Part print with two shaded views. Sizes in mm from the minimum x, y, z corner. A direction names the side the tool comes from. Give positions to 0.01 mm unless a question says otherwise; leave off trailing zeros. Loops run counter-clockwise (first coordinate to the right, second up) from the corner with the lowest first, then second, coordinate; pieces in that order, holes last. Notation, with made-up numbers: M 17.5,-7.5 L 47.5,-7.5 A26 cw 47.5,7.5 Z; hole C 47,86.25 d6. An arc over 180 degrees is marked long. Answer as a JSON object with one key per item and string values. Group by question number.
1. Slice it at B-B (z = 10). List the corners of the cut face in (x, y).
2. Drop flat-ended pins along their axis: pin 1 Ø10.5 at (y, z) = (3.5, 11) entering from -X; pin 2 Ø5.5 at (x, z) = (34, 9) entering from +Y; pin 3 Ø4 at (x, y) = (37.5, 17) entering from -Z. Give the stop position or say it passes through.
3. Slice it at C-C (x = 31). List the corners of the cut face in (y, z).
4. Mould opens along Y. For the marked faces 1, 2 and 3 say: released by +Y, released by -Y, zero draft, split by the parting line, or undercut.
5. Slice it at A-A (x = 25). List the corners of the cut face in (y, z).
6. Slice it at D-D (y = 17.75). List the corners of the cut face in (x, z), then the cut area to 3 significant figures.
7. 3-axis set-ups, long thin cutter, end or side, ignore diameter. For the marked faces 4, 5 and 6: which of +Z, -Z, +X, -X, +Y, -Y reach the whole face in a straight line?
8. Drill centre lines: line 1 along Y through (x, z) = (10, 26); line 2 along X through (y, z) = (3.4, 10); line 3 along Y through (x, z) = (20, 26). Where is each one in solid material? Low to high. Write a range as [from, to].
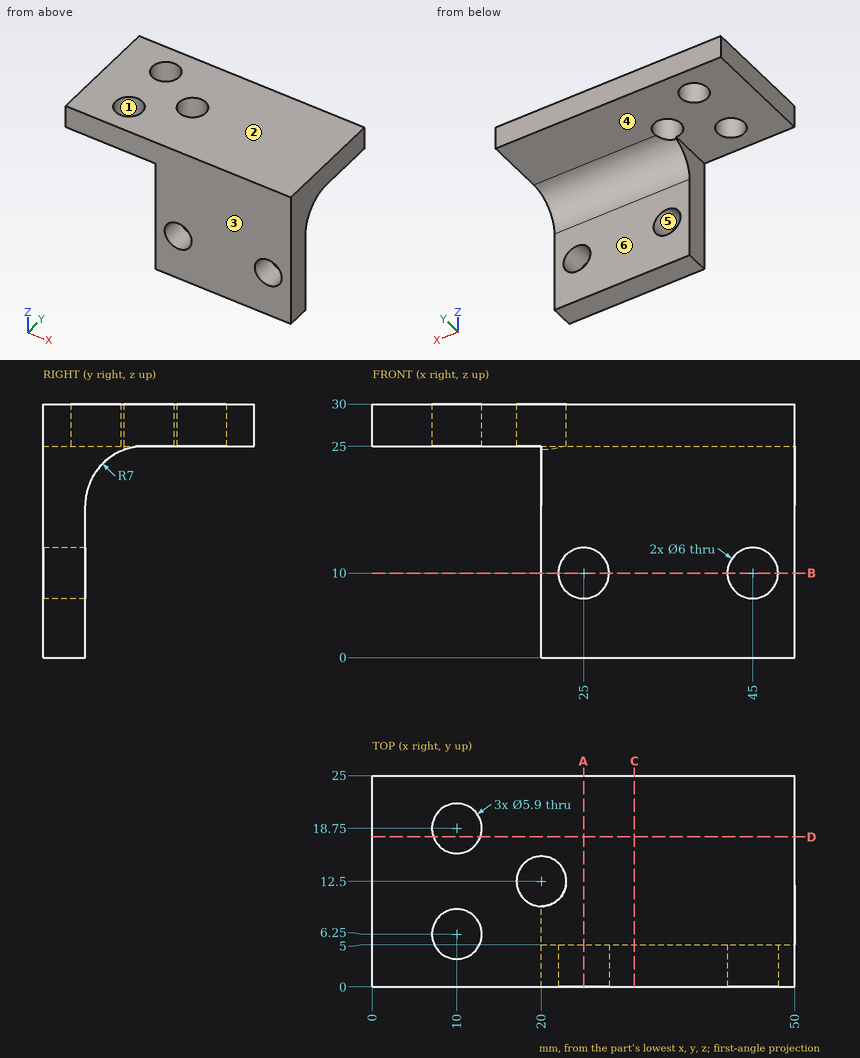
Established:
{
 "1": {"outline": "M 20,0 L 22,0 L 22,5 L 20,5 Z; M 28,0 L 42,0 L 42,5 L 28,5 Z; M 48,0 L 50,0 L 50,5 L 48,5 Z"},
 "2": {"pin 1": "stops at x = 20", "pin 2": "stops at y = 5", "pin 3": "stops at z = 25"},
 "3": {"outline": "M 0,0 L 5,0 L 5,18 A7 cw 12,25 L 25,25 L 25,30 L 0,30 Z"},
 "4": {"face 1": "undercut", "face 2": "zero draft", "face 3": "released by -Y"},
 "5": {"outline": "M 0,0 L 5,0 L 5,7 L 0,7 Z; M 0,13 L 5,13 L 5,18 A7 cw 12,25 L 25,25 L 25,30 L 0,30 Z"},
 "6": {"outline": "M 0,25 L 7.22,25 L 7.22,30 L 0,30 Z; M 12.78,25 L 50,25 L 50,30 L 12.78,30 Z", "area": "222 mm^2"},
 "7": {"face 4": "-Z, -X, +Y", "face 5": "+Y, -Y", "face 6": "-Z, +X, -X, +Y"},
 "8": {"line 1": "y = [0, 3.3], [9.2, 15.8], [21.7, 25]", "line 2": "x = [20, 22], [28, 42], [48, 50]", "line 3": "y = [0, 9.55], [15.45, 25]"}
}
